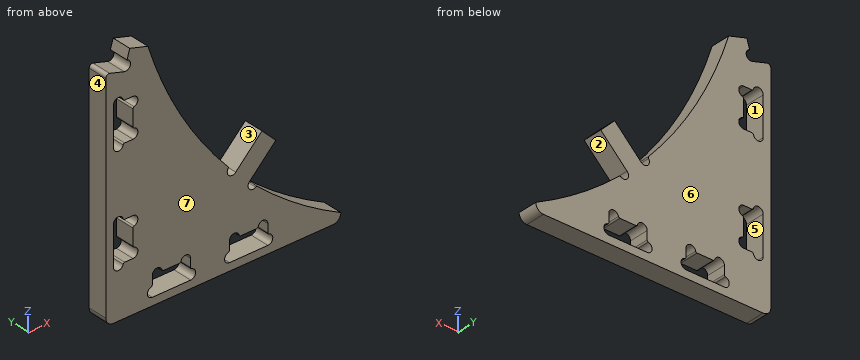
```python
from build123d import *

# Parameters (mm, degrees)
SKETCH1_W           = 25
SKETCH1_H           = 12.7
SKETCH1_W_2         = 12.7
SKETCH1_H_2         = 25
BOSS_EXTRUDE1_DEPTH = 12.7
SKETCH2_R           = 3.2
CUT_EXTRUDE1_DEPTH  = 351.503213473
FILLET1_R           = 5
FILLET2_R           = 1
FILLET3_R           = 2


with BuildPart() as part:
    # Sketch1 → Boss-Extrude1 (new body)
    with BuildSketch(Plane(origin=(0, 0, 0), x_dir=(1, 0, 0), z_dir=(0, 1, 0))):
        with BuildLine():
            Line((-172.193276216, 181.244243015), (-154.927095758, 163.978062557))
            Line((-154.927095758, 163.978062557), (-163.978062557, 154.927095758))
            Line((-163.978062557, 154.927095758), (-181.244243015, 172.193276216))
            ThreePointArc((-181.244243015, 172.193276216), (-215.239427447, 127.169134904), (-238.273429132, 75.668837508))
            Line((-238.273429132, 75.668837508), (-250.116468804, 72.111522519))
            Line((-250.116468804, 72.111522519), (-253.769935453, 84.27467102))
            Line((-253.769935453, 84.27467102), (-265.736660352, 80.680204478))
            Line((-265.736660352, 80.680204478), (-265.736660352, 228.2))
            Line((-265.736660352, 228.2), (-112.613320704, 228.2))
            Line((-112.613320704, 228.2), (-112.613320704, 223.2))
            ThreePointArc((-112.613320704, 223.2), (-143.940163951, 204.40457236), (-172.193276216, 181.244243015))
        make_face()
        with Locations((-172.656660352, 216.85)):
            Rectangle(SKETCH1_W, SKETCH1_H, mode=Mode.SUBTRACT)
        with Locations((-222.946660352, 216.85)):
            Rectangle(SKETCH1_W, SKETCH1_H, mode=Mode.SUBTRACT)
        with Locations((-254.386660352, 183)):
            Rectangle(SKETCH1_W_2, SKETCH1_H_2, mode=Mode.SUBTRACT)
        with Locations((-254.386660352, 113.474827547)):
            Rectangle(SKETCH1_W_2, SKETCH1_H_2, mode=Mode.SUBTRACT)
    extrude(amount=BOSS_EXTRUDE1_DEPTH)

    # Sketch2 → Cut-Extrude1 (cut, through all)
    with BuildSketch(Plane(origin=(0, 12.7, 0), x_dir=(1, 0, 0), z_dir=(0, 1, 0))):
        with Locations((-169.859291345, 183.433424282)):
            Circle(SKETCH2_R)
        with Locations((-183.433424282, 169.859291345)):
            Circle(SKETCH2_R)
        with Locations((-181.956660352, 210.5)):
            Circle(SKETCH2_R)
        with Locations((-163.356660352, 210.5)):
            Circle(SKETCH2_R)
        with Locations((-160.156660352, 220)):
            Circle(SKETCH2_R)
        with Locations((-185.156660352, 220)):
            Circle(SKETCH2_R)
        with Locations((-210.446660352, 220)):
            Circle(SKETCH2_R)
        with Locations((-213.646660352, 210.5)):
            Circle(SKETCH2_R)
        with Locations((-232.246660352, 210.5)):
            Circle(SKETCH2_R)
        with Locations((-235.446660352, 220)):
            Circle(SKETCH2_R)
        with Locations((-257.536660352, 195.5)):
            Circle(SKETCH2_R)
        with Locations((-248.036660352, 192.3)):
            Circle(SKETCH2_R)
        with Locations((-248.036660352, 173.7)):
            Circle(SKETCH2_R)
        with Locations((-257.536660352, 170.5)):
            Circle(SKETCH2_R)
        with Locations((-257.536660352, 125.974827547)):
            Circle(SKETCH2_R)
        with Locations((-257.536660352, 100.974827547)):
            Circle(SKETCH2_R)
        with Locations((-248.036660352, 104.174827547)):
            Circle(SKETCH2_R)
        with Locations((-248.036660352, 122.774827547)):
            Circle(SKETCH2_R)
        with Locations((-252.849376927, 81.209940689)):
            Circle(SKETCH2_R)
    extrude(amount=-CUT_EXTRUDE1_DEPTH, mode=Mode.SUBTRACT)

    # Fillet1
    fillet1_edges = [part.edges().sort_by_distance(p)[0] for p in [
        (-112.613320704, 6.35, -228.2),
        (-265.736660352, 6.35, -228.2),
    ]]
    fillet(fillet1_edges, radius=FILLET1_R - 0.0001)  # a hair under: the kernel refuses the full size

    # Fillet2
    fillet2_edges = [part.edges().sort_by_distance(p)[0] for p in [
        (-167.497476727, 6.35, -185.592551817),
        (-185.592551817, 6.35, -167.497476727),
        (-248.036660352, 6.35, -107.374827547),
        (-254.336660352, 6.35, -100.974827547),
        (-254.336660352, 6.35, -125.974827547),
        (-248.036660352, 6.35, -119.574827547),
        (-216.846660352, 6.35, -210.5),
        (-229.046660352, 6.35, -210.5),
        (-235.446660352, 6.35, -216.8),
        (-160.156660352, 6.35, -216.8),
        (-166.556660352, 6.35, -210.5),
        (-178.756660352, 6.35, -210.5),
        (-185.156660352, 6.35, -216.8),
        (-210.446660352, 6.35, -216.8),
        (-248.036660352, 6.35, -189.1),
        (-248.036660352, 6.35, -176.9),
        (-254.336660352, 6.35, -170.5),
        (-254.336660352, 6.35, -195.5),
    ]]
    fillet(fillet2_edges, radius=FILLET2_R)

    # Fillet3
    fillet3_edges = [part.edges().sort_by_distance(p)[0] for p in [
        (-265.736660352, 6.35, -80.680204478),
    ]]
    fillet(fillet3_edges, radius=FILLET3_R)


solid = part.part
```
Input: part model. Units: mm. Frame: model coordinates. Face numbers are marked on the shaded views. A direction names the side the tool comes from. Round coordinates to 2 decimals unless told otherwise and drop trailing zeros. Order: outer loops, then holes, each group sorted by start corner. A loop starts at its lowest first (then second) coordinate and runs counter-clockwise, first axis right, second up. Notation, with made-up numbers: (-26.5, 48) - (-15.5, 48) arc R16 cw to (-15.5, 64) - close; hole circle Ø8 at (-6, 71). An arc over 180 degrees is marked (long way). Answer in a Markdown table with one row per item.
Item 1: Section query C-C (x = -124.5). Return the cut outline in (y, z), then the cut area to 3 significant figures.
Model answer:
| item | result |
|---|---|
| outline | (0, -228.2) - (12.7, -228.2) - (12.7, -216.79) - (0, -216.79) - close |
| area | 145 mm² |
Item 2: Section query A-A (z = -162). Return the cut outline in (x, y).
Model answer:
| item | result |
|---|---|
| outline | (-265.74, 0) - (-190.41, 0) - (-190.41, 12.7) - (-265.74, 12.7) - close; (-171.05, 0) - (-156.91, 0) - (-156.91, 12.7) - (-171.05, 12.7) - close |
Item 3: Pin query (flat end, axial travel): pin 1 (4.5 mm diameter, centred on x = -252, y = 8.5, fed in from +Z); pin 2 (6 mm diameter, centred on x = -194, y = 6.5, fed in from +Z); pin 3 (4 mm diameter, centred on x = -174, y = 7, fed in from +Z). Return the tip coordinate at first contact, or that it passes through.
Model answer:
| item | result |
|---|---|
| pin 1 | stops at z = -72.11 |
| pin 2 | stops at z = -153.92 |
| pin 3 | stops at z = -162.95 |
Item 4: Mould query, pull axis Y, two halves, no side actions, for the marked faces 5, 6 and 7. Classes: released by +Y, released by -Y, zero draft, split by the parting line, or undercut.
Model answer:
| item | result |
|---|---|
| face 5 | zero draft |
| face 6 | released by +Y |
| face 7 | released by -Y |
Item 5: Section query B-B (x = -225.5). Return the cut outline in (y, z).
Model answer:
| item | result |
|---|---|
| outline | (0, -228.2) - (12.7, -228.2) - (12.7, -223.2) - (0, -223.2) - close; (0, -210.5) - (12.7, -210.5) - (12.7, -107.93) - (0, -107.93) - close |
Item 6: Line query: line 1 (Z direction, x = -220, y = 3.75); line 2 (Z direction, x = -254, y = 2.75); line 3 (Z direction, x = -171, y = 9.5). Output: solid intervals per line, ascending.
Model answer:
| item | result |
|---|---|
| line 1 | z = -228.2 to -223.2, -210.5 to -118.74 |
| line 2 | z = -228.2 to -195.66, -170.34 to -126.13, -100.81 to -84.21 |
| line 3 | z = -228.2 to -223.2, -210.5 to -186.42, -180.05 to -161.95 |
Item 7: Section query D-D (y = 5.5). Give the number of separate pieces and of enclosed holes in the cut face, then the cut area to 3 significant figures.
Model answer:
| item | result |
|---|---|
| separate pieces | 1 |
| enclosed holes | 4 |
| area | 10,200 mm² |
Item 8: Reachability of the marked faces 1, 2, 3 and 4 from +Z, -Z, +X, -X, +Y, -Y: full face, straight path, thin tool, end or side. Return the list, or none.
Model answer:
| item | result |
|---|---|
| face 1 | +Y, -Y |
| face 2 | +X, +Y, -Y |
| face 3 | +Z, +Y, -Y |
| face 4 | +Z, -Z, -X, +Y, -Y |
